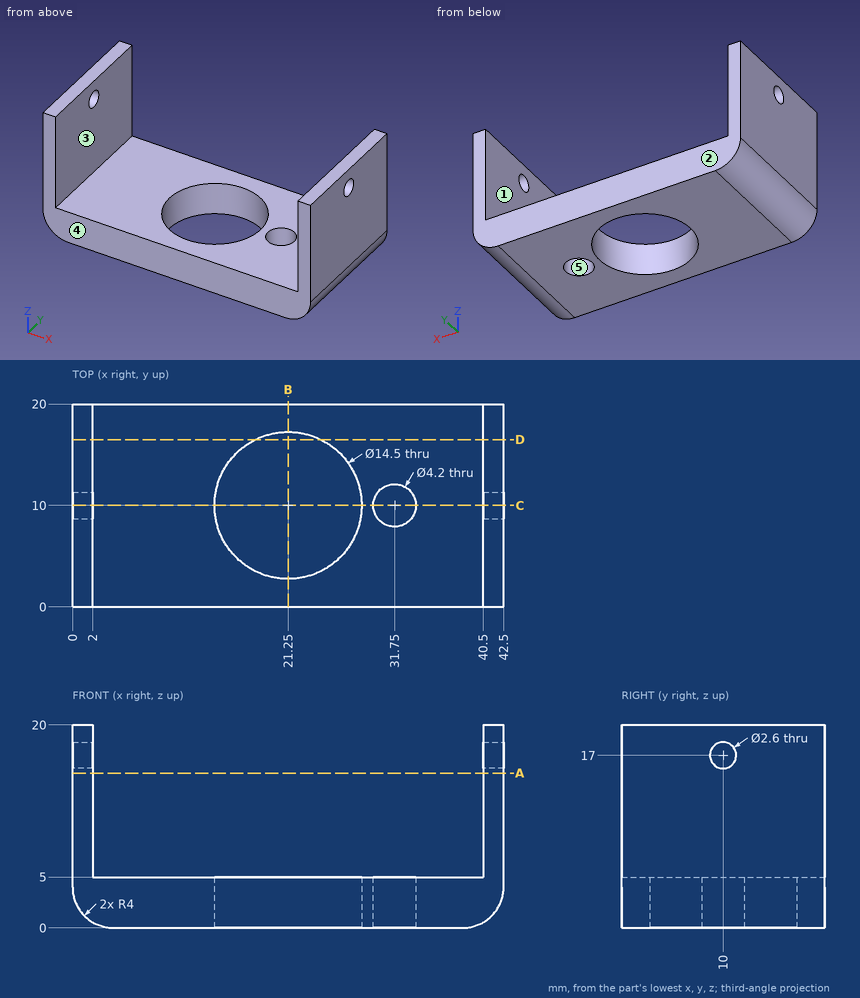
The drawing under review shows one solid part. Ordinate dimensions are in mm from its lowest x, y, z. A direction names the side the tool comes from. Coordinates: 2 decimals unless noted, no trailing zeros. Order: outer loops, then holes, each group sorted by start corner. A loop starts at its lowest first (then second) coordinate and runs counter-clockwise, first axis right, second up. Notation, with made-up numbers: (-15.5, -29) -> (-7.5, -29) arc R27 ccw to (-7.5, 5) -> close; hole circle Ø8 at (23, -17). An arc over 180 degrees is marked (long way). Use CSV: the item, a comma, the result in double quotes. Start each with the question number.
Item 1: We need section C-C, the plane y = 10. Give the boundary of the cut face in (x, z), then the cut area to 3 significant figures.
Item 2: We need section D-D, the plane y = 16.5. Give the boundary of the cut face in (x, z), then the cut area to 3 significant figures.
Item 3: For the marked faces 1 and 2, list the 3-axis set-ups (+Z, -Z, +X, -X, +Y, -Y) from which the entire face can be reached by the end or side of a thin tool; tool diameter is ignored.
Item 4: Wall thickness on probe 1 along X at (y, z) = (13.25, 11.75); probe 2 along Y at (x, z) = (21.25, 2.1); probe 3 along Y at (x, z) = (41.1, 17): over which ranges is each line inside the solid? List them lowest first.
Item 5: Insertion check: pin 1 (3 mm diameter, centred on y = 10, z = 17, fed in from +X); pin 2 (12 mm diameter, centred on x = 15, y = 2, fed in from +Z). Each pin has a flat end and moves straight along its axis. Give the tip position at first contact, or say it passes through.
Item 6: We need section A-A, the plane z = 15.25. Give the boundary of the cut face in (x, y).
Item 7: We need section B-B, the plane x = 21.25. Give the boundary of the cut face in (y, z).
Item 8: Draft analysis for pull direction Y (two halves, no side actions). For the marked faces 3, 4 and 5, state which applies: pulls with the +Y half, pulls with the -Y half, needs draft (parallel to the pull), parting line crosses it, or undercut.
Derived:
1,outline,"(0, 4) arc R4 ccw to (4, 0) -> (14, 0) -> (14, 5) -> (2, 5) -> (2, 15.7) -> (0, 15.7) -> close; (0, 18.3) -> (2, 18.3) -> (2, 20) -> (0, 20) -> close; (28.5, 0) -> (29.65, 0) -> (29.65, 5) -> (28.5, 5) -> close; (33.85, 0) -> (38.5, 0) arc R4 ccw to (42.5, 4) -> (42.5, 15.7) -> (40.5, 15.7) -> (40.5, 5) -> (33.85, 5) -> close; (40.5, 18.3) -> (42.5, 18.3) -> (42.5, 20) -> (40.5, 20) -> close"
1,area,"162 mm^2"
2,outline,"(0, 4) arc R4 ccw to (4, 0) -> (18.04, 0) -> (18.04, 5) -> (2, 5) -> (2, 20) -> (0, 20) -> close; (24.46, 0) -> (38.5, 0) arc R4 ccw to (42.5, 4) -> (42.5, 20) -> (40.5, 20) -> (40.5, 5) -> (24.46, 5) -> close"
2,area,"234 mm^2"
3,face 1,"+Z, +Y, -Y"
3,face 2,"+Z, -Z, +X, -X, +Y"
4,probe 1,"x = 0 to 2, 40.5 to 42.5"
4,probe 2,"y = 0 to 2.75, 17.25 to 20"
4,probe 3,"y = 0 to 8.7, 11.3 to 20"
5,pin 1,"stops at x = 42.5"
5,pin 2,"stops at z = 5"
6,outline,"(0, 0) -> (2, 0) -> (2, 20) -> (0, 20) -> close; (40.5, 0) -> (42.5, 0) -> (42.5, 20) -> (40.5, 20) -> close"
7,outline,"(0, 0) -> (2.75, 0) -> (2.75, 5) -> (0, 5) -> close; (17.25, 0) -> (20, 0) -> (20, 5) -> (17.25, 5) -> close"
8,face 3,"needs draft"
8,face 4,"pulls with the -Y half"
8,face 5,"undercut"
